Could you check a few things on this model? Use its own coordinates, in mm. Face numbers are marked on the shaded views. A direction names the side the tool comes from. Coordinates: 2 decimals unless noted, no trailing zeros. Write each loop counter-clockwise with the first axis right and the second up, starting at its lowest first coordinate (ties: lowest second). Pieces come first, ordered by that corner, then holes.
Item 1: For P1, Ø6, axis at x = 25, z = 25, coming from the -Y side; P2, Ø6.5, axis at x = -25, z = 0, coming from the -Y side; P3, Ø3, axis at y = 23.5, z = -19.5, coming from the +X side; P4, Ø6, axis at x = 11, y = 15.5, coming from the +Z side, each with a flat end and sliding along its axis, tell me the tip position at first contact or that it passes through.
Item 2: I want a section at A-A on x = 25. Please give me the cut outline in (y, z), then the cut area to 3 significant figures.
Item 3: Which directions (+Z, -Z, +X, -X, +Y, -Y) give clear straight access to the entire face, cutting with the end or side of a thin tool? Please do the marked faces 4, 5, 6 and 7.
Item 4: I want a section at B-B on z = 25. Please give me the cut outline in (x, y), then the cut area to 3 significant figures.
Item 5: If I drill on probe 1 along X at (y, z) = (7.5, 25); probe 2 along Z at (x, y) = (-25, 6.5), over which ranges is the centre line in solid material (lowest first)?
Item 6: I want a section at D-D on y = 14. Please give me the cut outline in (x, z), then the cut area to 3 significant figures.
Item 7: Thinking about a two-plate mould opening in Z: for the marked faces 1, 2 and 3, which applies, +Z half, -Z half, draft (parallel to the pull), parting line (faces both ways), or undercut?
Item 8: I want a section at C-C on y = 24.25. Please give me the cut outline in (x, z), then the cut area to 3 significant figures.
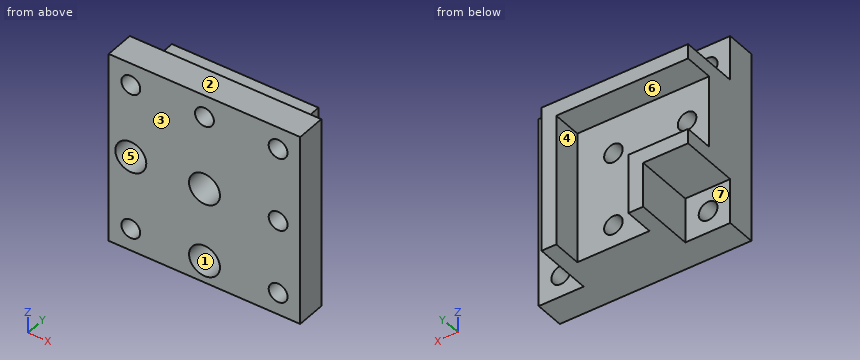
from build123d import *

# Parameters (mm, degrees)
SKETCH_1_W          = 65
SKETCH_1_H          = 65
SKETCH_1_R          = 3.2
EXTRUDE_1_DEPTH     = 10
EXTRUDE_3_DEPTH     = 10
SKETCH_4_R          = 5.25
CUT_EXTRUDE_1_DEPTH = 10
SKETCH_5_R          = 3.15
CUT_EXTRUDE_2_DEPTH = 20
EXTRUDE_4_DEPTH     = 20


with BuildPart() as part:
    # 스케치1 → 보스-돌출1 (new body)
    with BuildSketch(Plane(origin=(0, 0, 0), x_dir=(1, 0, 0), z_dir=(0, 1, 0))):
        Rectangle(SKETCH_1_W, SKETCH_1_H)
        with Locations((25, 0)):
            Circle(SKETCH_1_R, mode=Mode.SUBTRACT)
        with Locations((0, -25)):
            Circle(SKETCH_1_R, mode=Mode.SUBTRACT)
        with Locations((25, 25)):
            Circle(SKETCH_1_R, mode=Mode.SUBTRACT)
        with Locations((-25, 25)):
            Circle(SKETCH_1_R, mode=Mode.SUBTRACT)
        with Locations((25, -25)):
            Circle(SKETCH_1_R, mode=Mode.SUBTRACT)
        with Locations((-25, -25)):
            Circle(SKETCH_1_R, mode=Mode.SUBTRACT)
    extrude(amount=EXTRUDE_1_DEPTH)

    # 스케치2 → 보스-돌출3 (add)
    with BuildSketch(Plane(origin=(0, 10, 0), x_dir=(1, 0, 0), z_dir=(0, 1, 0))):
        Polygon((-32.5, -12.25), (12.25, -12.25), (12.25, 32.5), (-12.25, 32.5), (-12.25, 12.25), (-32.5, 12.25), align=None)
    extrude(amount=EXTRUDE_3_DEPTH)

    # 스케치4 → 컷-돌출1 (cut)
    with BuildSketch(Plane.XZ):
        Circle(SKETCH_4_R)
        with Locations((-25, 0)):
            Circle(SKETCH_4_R)
        with Locations((0, -25)):
            Circle(SKETCH_4_R)
    extrude(amount=-CUT_EXTRUDE_1_DEPTH, mode=Mode.SUBTRACT)

    # 스케치5 → 컷-돌출2 (cut)
    with BuildSketch(Plane.XZ):
        Circle(SKETCH_5_R)
        with Locations((0, -25)):
            Circle(SKETCH_5_R)
        with Locations((-25, 0)):
            Circle(SKETCH_5_R)
    extrude(amount=-CUT_EXTRUDE_2_DEPTH, mode=Mode.SUBTRACT)

    # 스케치6 → 보스-돌출4 (add)
    with BuildSketch(Plane(origin=(0, 10, 0), x_dir=(1, 0, 0), z_dir=(0, 1, 0))):
        Polygon((-12.25, 32.5), (-17.25, 32.5), (-17.25, 17.25), (-32.5, 17.25), (-32.5, 12.25), (-12.25, 12.25), align=None)
        Polygon((12.25, 32.5), (17.25, 32.5), (17.25, -17.25), (-32.5, -17.25), (-32.5, -12.25), (12.25, -12.25), align=None)
    extrude(amount=EXTRUDE_4_DEPTH)


solid = part.part
Response values:
1. P1: passes through
1. P2: stops at y = 10
1. P3: stops at x = 17.25
1. P4: stops at z = 17.25
2. outline: (0, -32.5) - (10, -32.5) - (10, -28.2) - (0, -28.2) - close; (0, -21.8) - (10, -21.8) - (10, -3.2) - (0, -3.2) - close; (0, 3.2) - (10, 3.2) - (10, 21.8) - (0, 21.8) - close; (0, 28.2) - (10, 28.2) - (10, 32.5) - (0, 32.5) - close
2. area: 458 mm2
3. face 4: -Z, +Y
3. face 5: -Y
3. face 6: -X, +Y
3. face 7: -Z, -X, +Y
4. outline: (-32.5, 0) - (-28.2, 0) - (-28.2, 10) - (-32.5, 10) - close; (-21.8, 0) - (-3.2, 0) - (-3.2, 10) - (-21.8, 10) - close; (3.2, 0) - (21.8, 0) - (21.8, 10) - (3.2, 10) - close; (28.2, 0) - (32.5, 0) - (32.5, 10) - (28.2, 10) - close
4. area: 458 mm2
5. probe 1: x = -32.5 to -28.2, -21.8 to -3.2, 3.2 to 21.8, 28.2 to 32.5
5. probe 2: z = -32.5 to -28.2, -21.8 to -5.25, 5.25 to 21.8, 28.2 to 32.5
6. outline: (-32.5, -17.25) - (-17.25, -17.25) - (-17.25, -32.5) - (17.25, -32.5) - (17.25, 17.25) - (-32.5, 17.25) - close; hole circle Ø6.3 at (-25, 0); hole circle Ø6.3 at (0, -25); hole circle Ø6.3 at (0, 0)
6. area: 2,150 mm2
7. face 1: undercut
7. face 2: +Z half
7. face 3: draft
8. outline: (-32.5, -17.25) - (-17.25, -17.25) - (-17.25, -32.5) - (-12.25, -32.5) - (-12.25, -12.25) - (-32.5, -12.25) - close; (-32.5, 12.25) - (12.25, 12.25) - (12.25, -32.5) - (17.25, -32.5) - (17.25, 17.25) - (-32.5, 17.25) - close
8. area: 650 mm2
